Part print with two shaded views. Sizes in mm from the minimum x, y, z corner. A direction names the side the tool comes from. Coordinates: 2 decimals unless noted, no trailing zeros. Write each loop counter-clockwise with the first axis right and the second up, starting at its lowest first coordinate (ties: lowest second). Pieces come first, ordered by that corner, then holes.
Q1. Drill centre lines: probe 1 along Z at (x, y) = (31, 0.75) (1 decimal); probe 2 along Z at (x, y) = (24, 0.85) (1 decimal); probe 3 along Z at (x, y) = (18, 1.9) (1 decimal). Where is each one in solid material? Low to high.
Q2. Pin check, flat tips, straight feed: P1, Ø1.3, axis at x = 10.5, y = 1.5, coming from the -Z side; P2, Ø0.8, axis at x = 30, y = 1.5, coming from the +Z side; P3, Ø0.8, axis at x = 29, y = 1.5, coming from the -Z side. Stop position of each tip, or through.
Q3. Band-saw the part on A-A, the plane y = 1.7. State how many separate pieces and enclosed holes the cut face has, plus the area to 3 significant figures.
Q4. Band-saw the part on B-B, the plane x = 7.5. Write the cut outline in (y, z).
Q5. Band-saw the part on C-C, the plane z = 17.78. Write the cut outline in (x, y).
Q6. Which spindle directions (+Z, -Z, +X, -X, +Y, -Y) get a long thin tool onto all of the face, cutting with end or side? Do the marked faces 1 and 2. Say none if no direction does.
Q7. Band-saw the part on D-D, the plane x = 27.5. Write the cut outline in (y, z) (1 decimal).
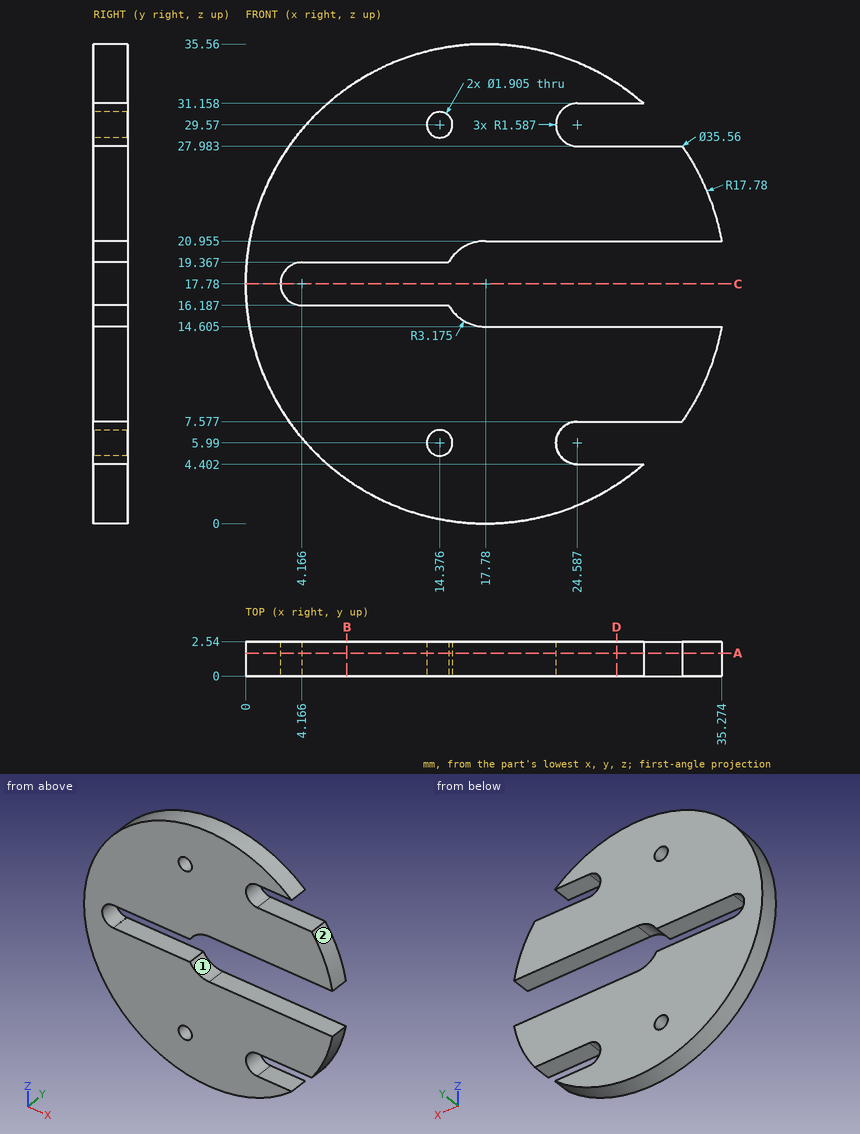
Answer sheet:
1. probe 1: z = 7.6 to 14.6, 21 to 28
1. probe 2: z = 1.1 to 4.5, 7.5 to 14.6, 21 to 28.1, 31 to 34.4
1. probe 3: z = 0 to 14.6, 21 to 35.6
2. P1: stops at z = 1.28
2. P2: stops at z = 27.98
2. P3: stops at z = 3.67
3. separate pieces: 1
3. enclosed holes: 2
3. area: 773 mm2
4. outline: (0, 3.27) - (2.54, 3.27) - (2.54, 16.19) - (0, 16.19) - close; (0, 19.37) - (2.54, 19.37) - (2.54, 32.29) - (0, 32.29) - close
5. outline: (0, 0) - (2.58, 0) - (2.58, 2.54) - (0, 2.54) - close
6. face 1: +X, +Y, -Y
6. face 2: +Z, +X, +Y, -Y
7. outline: (0, 2.9) - (2.5, 2.9) - (2.5, 4.4) - (0, 4.4) - close; (0, 7.6) - (2.5, 7.6) - (2.5, 14.6) - (0, 14.6) - close; (0, 21) - (2.5, 21) - (2.5, 28) - (0, 28) - close; (0, 31.2) - (2.5, 31.2) - (2.5, 32.7) - (0, 32.7) - close
